The listing builds one solid part. Answer for the finished solid, in the listing's coordinates (mm). A direction names the side the tool comes from. Round coordinates to 2 decimals unless told otherwise and drop trailing zeros. Order: outer loops, then holes, each group sorted by start corner. A loop starts at its lowest first (then second) coordinate and runs counter-clockwise, first axis right, second up. Notation, with made-up numbers: (62.5, 31.5) - (71.5, 31.5) arc R22 ccw to (71.5, 64.5) - close; hole circle Ø9 at (4, 18). An arc over 180 degrees is marked (long way). One line per item, written item: value. Start each with the question number.
1. A flat-ended cylindrical pin translates along its axis: P1, Ø4.5, axis at x = 20.62, y = 39, coming from the +Z side. Find the tip coordinate at first contact, or state that the pin passes through.
2. Section A-A, the plane y = 11 is taken. Give the vertices of the cut face in (x, z).
3. A tool of negligible diameter and unlimited length cuts with its end or side. For faces 1 (the flat face through (22, 40, 2.5)), 2 (the flat face through (12.622, 54, 2)), 3 (the flat face through (28, 40, 5)), from which of +Z, -Z, +X, -X, +Y, -Y can it reach the whole face along a straight path? Write none if from no direction.
4. Section B-B, the plane z = 1 is taken. Give the vertices of the cut face in (x, y), then the cut area to 3 significant figures.
5. Straight lines are drawn through the part: line 1 (X direction, y = 17, z = 2.1); line 2 (X direction, y = 43, z = 3.9); line 3 (X direction, y = 52.5, z = 4.6) (3 decimals). For each, find the intervals that lie inside material, in ascending order.
6. For a pull along Y with two mould halves and no side action, classify faces 4 (the flat face through (28, 40, 0)), 5 (the flat face through (9.622, 52, 2)) as released by +Y, released by -Y, zero draft, split by the parting line, or undercut.
7. Section C-C, the plane y = 39 is taken. Count the separate pieces of the cut face and the enclosed holes in it, then the cut area to 3 significant figures.
from build123d import *

# Parameters (mm, degrees)
BASE_W                          = 50
BASE_H                          = 130
BASE_R                          = 14
BOSS_EXTRUDE1_DEPTH             = 5
CBORE_FOR_M2_5_SHCS1_AT_2_COUNT = 2
CBORE_FOR_M2_5_SHCS1_AT_2_PITCH = 15
FILLET3_R                       = 2
FILLET5_R                       = 3


with BuildPart() as part:
    # Base → Boss-Extrude1 (new body)
    with BuildSketch(Plane.XY):
        with Locations((28.12242927, 52.845785243)):
            Rectangle(BASE_W, BASE_H)
        with Locations((28.12242927, 59.845785243)):
            Circle(BASE_R, mode=Mode.SUBTRACT)
        with BuildLine():
            Line((46.62242927, 109.845785243), (46.62242927, -4.154214757))
            ThreePointArc((46.62242927, -4.154214757), (45.12242927, -5.654214757), (43.62242927, -4.154214757))
            Line((43.62242927, -4.154214757), (43.62242927, 109.845785243))
            ThreePointArc((43.62242927, 109.845785243), (45.12242927, 111.345785243), (46.62242927, 109.845785243))
        make_face(mode=Mode.SUBTRACT)
        with BuildLine():
            Line((12.62242927, 109.845785243), (12.62242927, -4.154214757))
            ThreePointArc((12.62242927, -4.154214757), (11.12242927, -5.654214757), (9.62242927, -4.154214757))
            Line((9.62242927, -4.154214757), (9.62242927, 109.845785243))
            ThreePointArc((9.62242927, 109.845785243), (11.12242927, 111.345785243), (12.62242927, 109.845785243))
        make_face(mode=Mode.SUBTRACT)
    extrude(amount=BOSS_EXTRUDE1_DEPTH)

    # Sketch5 → CBORE for M2.5 SHCS1 (revolve, cut)
    with BuildSketch(Plane(origin=(20.62242927, 38.995785243, 5), x_dir=(0, -1, 0), z_dir=(1, 0, 0))):
        Polygon((0, 0), (0, 5), (1.45, 5), (1.45, 2.525), (1.475, 2.5), (2.75, 2.5), (2.75, 0), align=None)
    cbore_for_m2_5_shcs1 = revolve(axis=Axis((20.62242927, 38.995785243, 11.35), (0, 0, -1)), mode=Mode.SUBTRACT)

    # CBORE for M2.5 SHCS1 at 2: CBORE for M2.5 SHCS1 ×2
    with Locations(*[(i * CBORE_FOR_M2_5_SHCS1_AT_2_PITCH, 0, 0) for i in range(1, CBORE_FOR_M2_5_SHCS1_AT_2_COUNT)]):
        add(cbore_for_m2_5_shcs1, mode=Mode.SUBTRACT)

    # Fillet3
    fillet3_edges = [part.edges().sort_by_distance(p)[0] for p in [
        (53.12242927, 52.845785243, 5),
        (28.12242927, 117.845785243, 5),
        (3.12242927, 52.845785243, 5),
        (28.12242927, 117.845785243, 0),
        (53.12242927, 52.845785243, 0),
        (28.12242927, -12.154214757, 0),
        (3.12242927, 52.845785243, 0),
        (28.12242927, -12.154214757, 5),
        (3.12242927, 117.845785243, 2.5),
        (53.12242927, 117.845785243, 2.5),
        (53.12242927, -12.154214757, 2.5),
        (3.12242927, -12.154214757, 2.5),
    ]]
    fillet(fillet3_edges, radius=FILLET3_R)

    # Fillet5
    # the kernel refuses this fillet: 3 mm, written as the material it takes off along each edge
    with BuildSketch(Plane(origin=(28.12242927, 59.845785243, 5), x_dir=(1, 0, 0), z_dir=(0, -1, 0))) as fillet5_piece_1:
        with BuildLine():
            CenterArc((14 + FILLET5_R, -FILLET5_R), FILLET5_R, 90, 90)
            Line((14, -FILLET5_R), (14, 0))
            Line((14, 0), (14 + FILLET5_R, 0))
        make_face()
    revolve(axis=Axis((28.12242927, 59.845785243, 5), (0, 0, 1)), mode=Mode.SUBTRACT)


solid = part.part
Answer list:
1. P1: stops at z = 2.5
2. outline: (3.12, 2) arc R2 ccw to (5.12, 0) - (9.62, 0) - (9.62, 5) - (5.12, 5) arc R2 ccw to (3.12, 3) - close; (12.62, 0) - (43.62, 0) - (43.62, 5) - (12.62, 5) - close; (46.62, 0) - (51.12, 0) arc R2 ccw to (53.12, 2) - (53.12, 3) arc R2 ccw to (51.12, 5) - (46.62, 5) - close
3. face 1: +Z
3. face 2: +Z, -Z
3. face 3: +Z, +X, -X, +Y, -Y
4. outline: (3.39, -10.15) arc R1.73 ccw to (5.12, -11.89) - (51.12, -11.89) arc R1.73 ccw to (52.85, -10.15) - (52.85, 115.85) arc R1.73 ccw to (51.12, 117.58) - (5.12, 117.58) arc R1.73 ccw to (3.39, 115.85) - close; hole (9.62, -4.15) arc R1.5 ccw to (12.62, -4.15) - (12.62, 109.85) arc R1.5 ccw to (9.62, 109.85) - close; hole circle Ø28 at (28.12, 59.85); hole circle Ø2.9 at (20.62, 39); hole circle Ø2.9 at (35.62, 39); hole (43.62, -4.15) arc R1.5 ccw to (46.62, -4.15) - (46.62, 109.85) arc R1.5 ccw to (43.62, 109.85) - close
4. area: 5,070 mm²
5. line 1: x = 3.12 to 9.62, 12.62 to 43.62, 46.62 to 53.12
5. line 2: x = 3.34 to 9.62, 12.62 to 43.62, 46.62 to 52.91
5. line 3: x = 3.922 to 9.622, 12.622 to 14.47, 41.775 to 43.622, 46.622 to 52.322
6. face 4: zero draft
6. face 5: undercut
7. separate pieces: 5
7. enclosed holes: 0
7. area: 175 mm²
